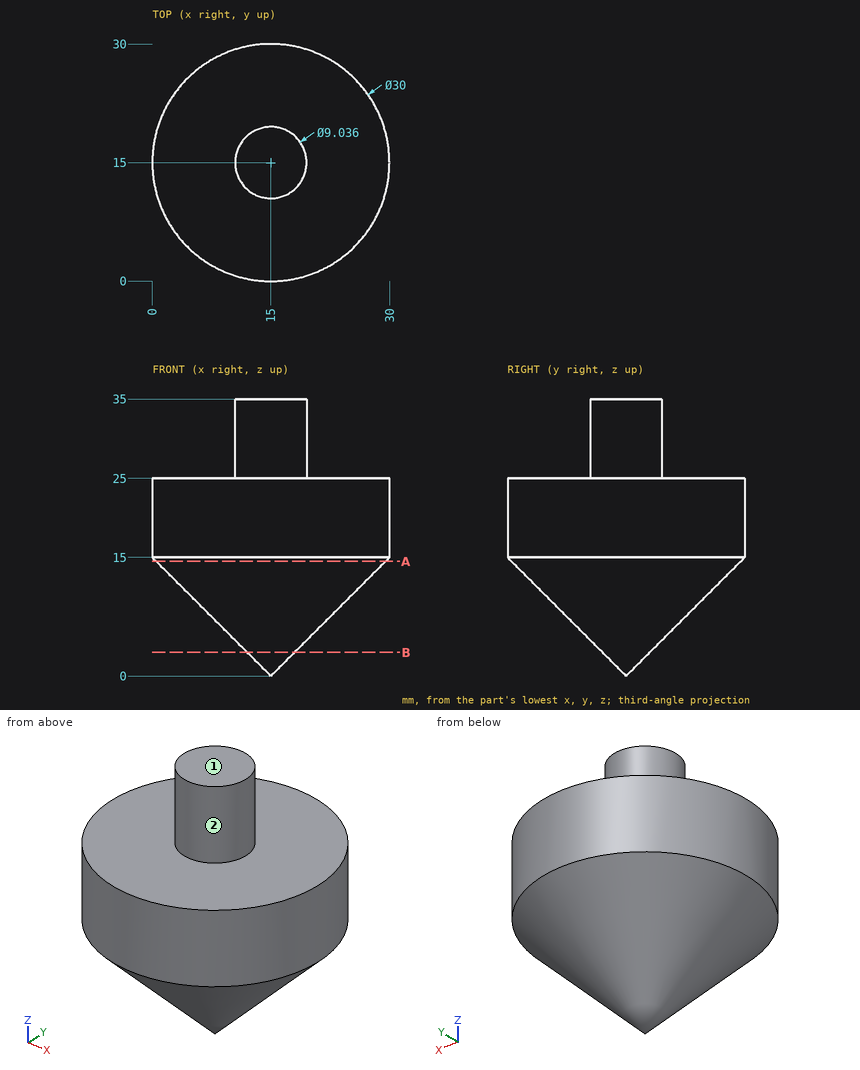
Part print with two shaded views. Sizes in mm from the minimum x, y, z corner. A direction names the side the tool comes from. Coordinates: 2 decimals unless noted, no trailing zeros. Write each loop counter-clockwise with the first axis right and the second up, starting at its lowest first coordinate (ties: lowest second). Pieces come first, ordered by that corner, then holes. Notation, with made-up numbers: M 76.25,35 L 126.25,35 A24 ccw 126.25,69 Z; hole C -27,70 d6. An arc over 180 degrees is marked long. Return JSON: item names as keys, results as strings.
Item 1: Slice it at A-A, the plane z = 14.5. Write the cut outline in (x, y).
Findings below:
{"outline": "C 15,15 d29"}
Item 2: Drop flat-ended pins along their axis: pin 1 Ø3 at (y, z) = (14, 14.5) entering from +X; pin 2 Ø1 at (x, z) = (5, 13) entering from -Y; pin 3 Ø4 at (x, z) = (9, 15) entering from +Y; pin 4 Ø2 at (y, z) = (12, 22) entering from -X. Give the stop position or say it passes through.
Findings below:
{"pin 1": "stops at x = 30", "pin 2": "stops at y = 5.75", "pin 3": "stops at y = 29.46", "pin 4": "stops at x = 0.13"}
Item 3: Slice it at B-B, the plane z = 3. Write the cut outline in (x, y).
Findings below:
{"outline": "C 15,15 d6"}
Item 4: Which spindle directions (+Z, -Z, +X, -X, +Y, -Y) get a long thin tool onto all of the face, cutting with end or side? Do the marked faces 1 and 2. Say none if no direction does.
Findings below:
{"face 1": "+Z, +X, -X, +Y, -Y", "face 2": "+Z"}
Item 5: Probe line 1 (Y direction, x = 14.75, z = 27); line 2 (Z direction, x = 21.5, y = 6.5); line 3 (X direction, y = 11.5, z = 14.5). List the from-to ranges inside material, lowest first. Write a range as from..to.
Findings below:
{"line 1": "y = 10.49..19.51", "line 2": "z = 10.7..25", "line 3": "x = 0.93..29.07"}
